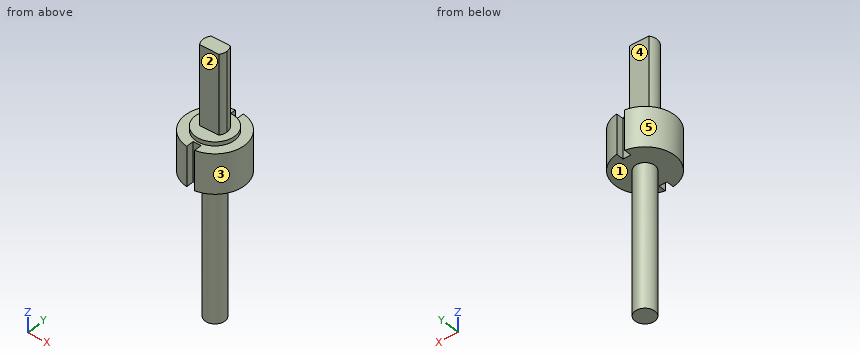
from build123d import *

# Parameters (mm, degrees)
SKETCH_1_R          = 7.5
EXTRUDE_1_DEPTH     = 5
SKETCH_6_R          = 5
EXTRUDE_6_DEPTH     = 1
EXTRUDE_7_DEPTH     = 20
SKETCH_9_R          = 2.5
EXTRUDE_8_DEPTH     = 36
SKETCH_11_W         = 2
SKETCH_11_H         = 2
CUT_EXTRUDE_1_DEPTH = 10


with BuildPart() as part:
    # Эскиз1 → Бобышка-Вытянуть1 (new, symmetric)
    with BuildSketch(Plane.XY):
        Circle(SKETCH_1_R)
    extrude(amount=EXTRUDE_1_DEPTH, both=True)

    # Эскиз6 → Бобышка-Вытянуть6 (add)
    with BuildSketch(Plane.XY.offset(5)):
        Circle(SKETCH_6_R)
    extrude(amount=EXTRUDE_6_DEPTH)

    # Эскиз10 → Бобышка-Вытянуть7 (add)
    with BuildSketch(Plane.XY.offset(6)):
        with BuildLine():
            Line((2.436698586, 1.75), (-2.436698586, 1.75))
            ThreePointArc((-2.436698586, 1.75), (-3, 0), (-2.436698586, -1.75))
            Line((-2.436698586, -1.75), (2.436698586, -1.75))
            ThreePointArc((2.436698586, -1.75), (2.855704445, -0.919212772), (3, 0))
            ThreePointArc((3, 0), (2.855704445, 0.919212772), (2.436698586, 1.75))
        make_face()
    extrude(amount=EXTRUDE_7_DEPTH)

    # Эскиз9 → Бобышка-Вытянуть8 (add)
    with BuildSketch(Plane(origin=(0, 0, -5), x_dir=(-1, 0, 0), z_dir=(0, 0, -1))):
        with Locations(Location((0, 0, 0), (0, 0, 180))):
            Circle(SKETCH_9_R)
    extrude(amount=EXTRUDE_8_DEPTH)

    # Эскиз11 → Вырез-Вытянуть1 (cut)
    with BuildSketch(Plane.XY.offset(5)):
        with Locations((0, 6.5)):
            Rectangle(SKETCH_11_W, SKETCH_11_H)
        with Locations((0, -6.5)):
            Rectangle(SKETCH_11_W, SKETCH_11_H)
    extrude(amount=-CUT_EXTRUDE_1_DEPTH, mode=Mode.SUBTRACT)


solid = part.part
Design review of the part built by this model. Coordinates are the model's own, in mm. Face numbers are marked on the shaded views. A direction names the side the tool comes from. Round coordinates to 2 decimals unless told otherwise and drop trailing zeros. Order: outer loops, then holes, each group sorted by start corner. A loop starts at its lowest first (then second) coordinate and runs counter-clockwise, first axis right, second up.
1) Machinability: for the marked faces 1, 2, 3, 4 and 5, which of the approach directions +Z, -Z, +X, -X, +Y, -Y give a long, thin tool a straight path to every point of the face, cutting with its end or side? Answer none if there is none.
The answers:
face 1: -Z
face 2: +Z, +X, -X, -Y
face 3: +Z, -Z, +X
face 4: +Z, +X, -X, +Y
face 5: +Z, -Z, -X
2) Clearance check with flat-ended pins moving along their axes: pin 1 Ø2 at (y, z) = (6.5, 2) entering from -X; pin 2 Ø1 at (x, y) = (-4.5, 2) entering from +Z; pin 3 Ø6 at (x, z) = (0.5, 15) entering from -Y. State where each tip first meets the part, or that it passes through.
The answers:
pin 1: stops at x = -5.1
pin 2: stops at z = 6
pin 3: stops at y = -1.75
3) Consider section B-B (z = 19.5). State the section outline as (x, y) points, plus the area to 3 significant figures.
The answers:
outline: (-2.44, -1.75) - (2.44, -1.75) arc R3 ccw to (2.44, 1.75) - (-2.44, 1.75) arc R3 ccw to start
area: 19.7 mm2
4) For L1, parallel to Z at x = 2.75, y = 4.75; L2, parallel to X at y = -0.5, z = -35; L3, parallel to Y at x = -0.75, z = 21.5, list the stretches that pass through material, from the lowest coordinate up.
The answers:
L1: z = -5 to 5
L2: x = -2.45 to 2.45
L3: y = -1.75 to 1.75
5) Consider section D-D (x = 6). State the section outline as (y, z) points, plus the area to 3 significant figures.
The answers:
outline: (-4.5, -5) - (4.5, -5) - (4.5, 5) - (-4.5, 5) - close
area: 90.0 mm2
6) Consider section C-C (y = -0.75). State the section outline as (x, z) points.
The answers:
outline: (-7.46, -5) - (-2.38, -5) - (-2.38, -41) - (2.38, -41) - (2.38, -5) - (7.46, -5) - (7.46, 5) - (4.94, 5) - (4.94, 6) - (2.9, 6) - (2.9, 26) - (-2.9, 26) - (-2.9, 6) - (-4.94, 6) - (-4.94, 5) - (-7.46, 5) - close
